```python
from build123d import *

# Parameters (mm, degrees)
SKETCH1_R                = 38.1
BOSS_EXTRUDE1_DEPTH      = 25.4
BOSS_EXTRUDE2_DEPTH      = 25.4
BOSS_EXTRUDE2_DEPTH_BACK = 25.4
BOSS_EXTRUDE3_DEPTH      = 88.9
BOSS_EXTRUDE3_DEPTH_BACK = 88.9
SKETCH4_R                = 254
FILLET1_R                = 25.4


with BuildPart() as part:
    # Sketch1 → Boss-Extrude1 (new body)
    with BuildSketch(Plane(origin=(0, 0, 0), x_dir=(1, 0, 0), z_dir=(0, 1, 0))):
        with BuildLine():
            Line((-514.35, 223.52), (514.35, 223.52))
            ThreePointArc((514.35, 223.52), (541.290768363, 212.360768363), (552.45, 185.42))
            Line((552.45, 185.42), (552.45, -185.42))
            ThreePointArc((552.45, -185.42), (541.290768363, -212.360768363), (514.35, -223.52))
            Line((514.35, -223.52), (-514.35, -223.52))
            ThreePointArc((-514.35, -223.52), (-541.290768363, -212.360768363), (-552.45, -185.42))
            Line((-552.45, -185.42), (-552.45, 185.42))
            ThreePointArc((-552.45, 185.42), (-541.290768363, 212.360768363), (-514.35, 223.52))
        make_face()
        with Locations(Location((-488.95, 160.02, 0), (0, 0, 270))):
            Circle(SKETCH1_R, mode=Mode.SUBTRACT)
        with Locations(Location((488.95, 160.02, 0), (0, 0, 270))):
            Circle(SKETCH1_R, mode=Mode.SUBTRACT)
        with Locations(Location((488.95, -160.02, 0), (0, 0, 270))):
            Circle(SKETCH1_R, mode=Mode.SUBTRACT)
        with Locations(Location((-488.95, -160.02, 0), (0, 0, 270))):
            Circle(SKETCH1_R, mode=Mode.SUBTRACT)
    extrude(amount=BOSS_EXTRUDE1_DEPTH)

    # Sketch3 → Boss-Extrude2 (add, two sides: drawn at the far end of the back side and taken through both)
    with BuildSketch(Plane.XY.offset(-BOSS_EXTRUDE2_DEPTH_BACK)):
        with BuildLine():
            Line((-190.5, 25.4), (190.5, 25.4))
            Line((190.5, 25.4), (190.5, 127))
            ThreePointArc((190.5, 127), (0, 41.005208253), (-190.5, 127))
            Line((-190.5, 127), (-190.5, 25.4))
        make_face()
    extrude(amount=BOSS_EXTRUDE2_DEPTH + BOSS_EXTRUDE2_DEPTH_BACK)

    # Sketch4 → Boss-Extrude3 (add, two sides: drawn at the far end of the back side and taken through both)
    with BuildSketch(Plane.XY.offset(-BOSS_EXTRUDE3_DEPTH_BACK)):
        with Locations((0, 295.005208253)):
            Circle(SKETCH4_R)
    extrude(amount=BOSS_EXTRUDE3_DEPTH + BOSS_EXTRUDE3_DEPTH_BACK)

    # Fillet1
    fillet1_edges = [part.edges().sort_by_distance(p)[0] for p in [
        (-254, 295.005208253, -88.9),
        (-254, 295.005208253, 88.9),
    ]]
    fillet(fillet1_edges, radius=FILLET1_R)


solid = part.part
```
Source: CAD feature listing. Evaluate the final solid. Frame: model axes, mm. A direction names the side the tool comes from. Give positions to 0.01 mm unless a question says otherwise; leave off trailing zeros. Loops run counter-clockwise (first coordinate to the right, second up) from the corner with the lowest first, then second, coordinate; pieces in that order, holes last. Notation, with made-up numbers: (30, 19.25) -> (68, 19.25) arc R10 ccw to (68, 31.25) -> close; hole circle Ø5 at (-2.75, -1.75). An arc over 180 degrees is marked (long way). Use a Markdown table: item, result. Add a question column.
(1) Section query A-A (z = 160.02). Output: boundary loops of the cut face in (x, y), then the cut area to 3 significant figures.
(2) Section query B-B (x = 0). Output: boundary loops of the cut face in (y, z).
(3) Pull-direction query (Y, two-part tool) for faces 6 (the face through (190.5, 75, 0)), 7 (the face through (540.99, 12.52, -212.66)), 8 (the face through (8, 0, -3)); classes: +Y half, -Y half, draft (parallel to the pull), parting line (faces both ways), or undercut.
(4) Access query for faces 1 (the face through (-3, 32, -25.4)), 2 (the face through (-190.5, 77, 0)), 3 (the face through (-3, 298, 88.9)), 4 (the face through (-3, 298, -88.9)), 5 (the face through (-3, 32, 25.4)). Directions: +Z, -Z, +X, -X, +Y, -Y. A direction counts if a zero-diameter tool reaches every point of the face in a straight line with its end or side. Return the directions, or none.
(5) Ray query, line 1 (X direction, y = 9, z = -160.02); line 2 (Z direction, x = -488, y = 16); line 3 (Y direction, x = -415, z = -112.5). Return the intervals inside material, ascending.
(6) First-contact query: pin 1 Ø6 at (y, z) = (240, -27.5) entering from -X; pin 2 Ø15 at (y, z) = (91.5, -11) entering from -X; pin 3 Ø6 at (x, z) = (-107.5, 53) entering from +Y. Flat tips, straight axial feed; report the tip coordinate or a pass-through.
(7) Section query C-C (x = 488.95). Output: boundary loops of the cut face in (y, z).
(8) Section query D-D (z = -45). Output: boundary loops of the cut face in (x, y).
Checked values:
| question | item | result |
|---|---|---|
| 1 | outline | (-552.45, 0) -> (-527.05, 0) -> (-527.05, 25.4) -> (-552.45, 25.4) -> close; (-450.85, 0) -> (450.85, 0) -> (450.85, 25.4) -> (-450.85, 25.4) -> close; (527.05, 0) -> (552.45, 0) -> (552.45, 25.4) -> (527.05, 25.4) -> close |
| 1 | area | 24,200 mm^2 |
| 2 | outline | (0, -223.52) -> (25.4, -223.52) -> (25.4, -25.4) -> (41.01, -25.4) -> (41.01, -63.5) arc R25.4 ccw to (66.41, -88.9) -> (523.61, -88.9) arc R25.4 ccw to (549.01, -63.5) -> (549.01, 63.5) arc R25.4 ccw to (523.61, 88.9) -> (66.41, 88.9) arc R25.4 ccw to (41.01, 63.5) -> (41.01, 25.4) -> (25.4, 25.4) -> (25.4, 223.52) -> (0, 223.52) -> close |
| 3 | face 6 | undercut |
| 3 | face 7 | draft |
| 3 | face 8 | -Y half |
| 4 | face 1 | -Z |
| 4 | face 2 | +Z, -Z, -X |
| 4 | face 3 | +Z, +X, -X, +Y |
| 4 | face 4 | -Z, +X, -X, +Y |
| 4 | face 5 | +Z |
| 5 | line 1 | -552.45 to -527.05, -450.85 to 450.85, 527.05 to 552.45 |
| 5 | line 2 | -223.52 to -198.11, -121.93 to 121.93, 198.11 to 223.52 |
| 5 | line 3 | 0 to 25.4 |
| 6 | pin 1 | x = -248.62 |
| 6 | pin 2 | x = -190.5 |
| 6 | pin 3 | y = 526.51 |
| 7 | outline | (0, -223.52) -> (25.4, -223.52) -> (25.4, -198.12) -> (0, -198.12) -> close; (0, -121.92) -> (25.4, -121.92) -> (25.4, 121.92) -> (0, 121.92) -> close; (0, 198.12) -> (25.4, 198.12) -> (25.4, 223.52) -> (0, 223.52) -> close |
| 8 | outline | (-552.45, 0) -> (552.45, 0) -> (552.45, 25.4) -> (-552.45, 25.4) -> close; circle Ø508 at (0, 295.01) |
